The model under review builds one solid part; all positions refer to its coordinate system, in mm. Face numbers are marked on the shaded views. A direction names the side the tool comes from. Round coordinates to 2 decimals unless told otherwise and drop trailing zeros. Order: outer loops, then holes, each group sorted by start corner. A loop starts at its lowest first (then second) coordinate and runs counter-clockwise, first axis right, second up. Notation, with made-up numbers: (-20.75, 41) -> (-3.75, 41) arc R18 cw to (-3.75, 63) -> close; hole circle Ø9 at (-11, 45.5). An arc over 180 degrees is marked (long way). Return JSON: item names as keys, results as strings. Group by question number.
from build123d import *

# Parameters (mm, degrees)
F0_R     = 26.5
F1_DEPTH = 100
F2_T     = -3
F3_R     = 75
F4_DEPTH = 3
F5_W     = 400
F5_H     = 400
F6_DEPTH = 16


# Not quite as in the source:
# - a feature names something its author has since deleted; it is built from what else it names


with BuildPart() as f1:
    # F0 (on Top) → F1 (new body)
    with BuildSketch(Plane.XY):
        Circle(F0_R)
    extrude(amount=F1_DEPTH)

    # F2
    f2_openings = [f1.faces().sort_by_distance(p)[0] for p in [
        (0, 0, 100),
        (0, 0, 0),
    ]]
    offset(amount=F2_T, openings=f2_openings)

    # F3 (on Top) → F4 (join)
    with BuildSketch(Plane.XY):
        Circle(F3_R)
    extrude(amount=F4_DEPTH)

    # F5 (on Top) → F6 (join)
    with BuildSketch(Plane.XY):
        with Locations((125, 125)):
            Rectangle(F5_W, F5_H)
    extrude(amount=-F6_DEPTH)


solid = f1.part
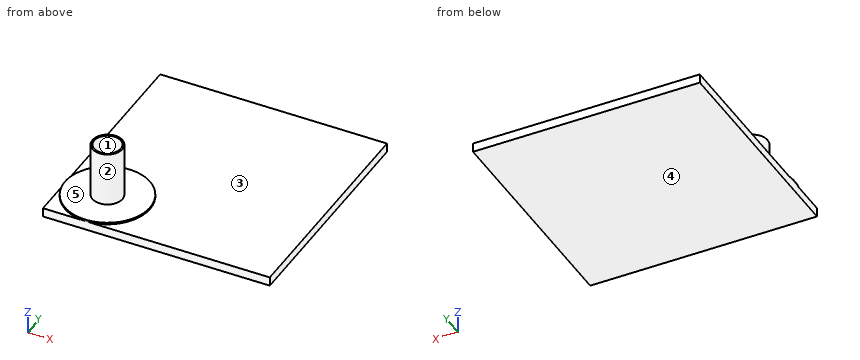
Item 1: For the marked faces 4 and 5, list the 3-axis set-ups (+Z, -Z, +X, -X, +Y, -Y) from which the entire face can be reached by the end or side of a thin tool; tool diameter is ignored.
Item 2: The part is to be moulded in two halves that separate along X. For the marked faces 1, 2 and 3, say which applies: +X half, -X half, draft (parallel to the pull), parting line (faces both ways), or undercut.
Item 3: Consider section B-B on x = 70. State the section outline as (y, z) points.
Item 4: Insertion check: pin 1 Ø3 at (y, z) = (-16, 67) entering from -X; pin 2 Ø4 at (x, z) = (-21, 6.5) entering from +Y; pin 3 Ø12 at (x, y) = (126.5, 75) entering from +Z. Each pin has a flat end and moves straight along its axis. Give the tip position at first contact, or say it passes through.
Item 5: Consider section D-D on x = 258. State the section outline as (y, z) points.
Item 6: Consider section A-A on y = 60. State the section outline as (x, z) points.
Item 7: Wall thickness on line 1 along X through (y, z) = (0, 67); line 2 along Z through (x, y) = (9.5, 105.5): over which ranges is each line inside the solid? List them lowest first.
Item 8: Consider section C-C on z = 79.5. State the section outline as (x, y) points, plus the area to 3 significant figures.
Values:
{
 "1": {"face 4": "-Z, +X, -X, +Y, -Y", "face 5": "+Z"},
 "2": {"face 1": "undercut", "face 2": "parting line", "face 3": "draft"},
 "3": {"outline": "(-75, -16) -> (325, -16) -> (325, 0) -> (26.93, 0) -> (26.93, 3) -> (-26.93, 3) -> (-26.93, 0) -> (-75, 0) -> close"},
 "4": {"pin 1": "x = -22.18", "pin 2": "y = 18.47", "pin 3": "z = 0"},
 "5": {"outline": "(-75, -16) -> (325, -16) -> (325, 0) -> (-75, 0) -> close"},
 "6": {"outline": "(-75, -16) -> (325, -16) -> (325, 0) -> (45, 0) -> (45, 3) -> (-45, 3) -> (-45, 0) -> (-75, 0) -> close"},
 "7": {"line 1": "-26.5 to -23.5, 23.5 to 26.5", "line 2": "-16 to 0"},
 "8": {"outline": "circle Ø53 at (0, 0); hole circle Ø47 at (0, 0)", "area": "471 mm^2"}
}
